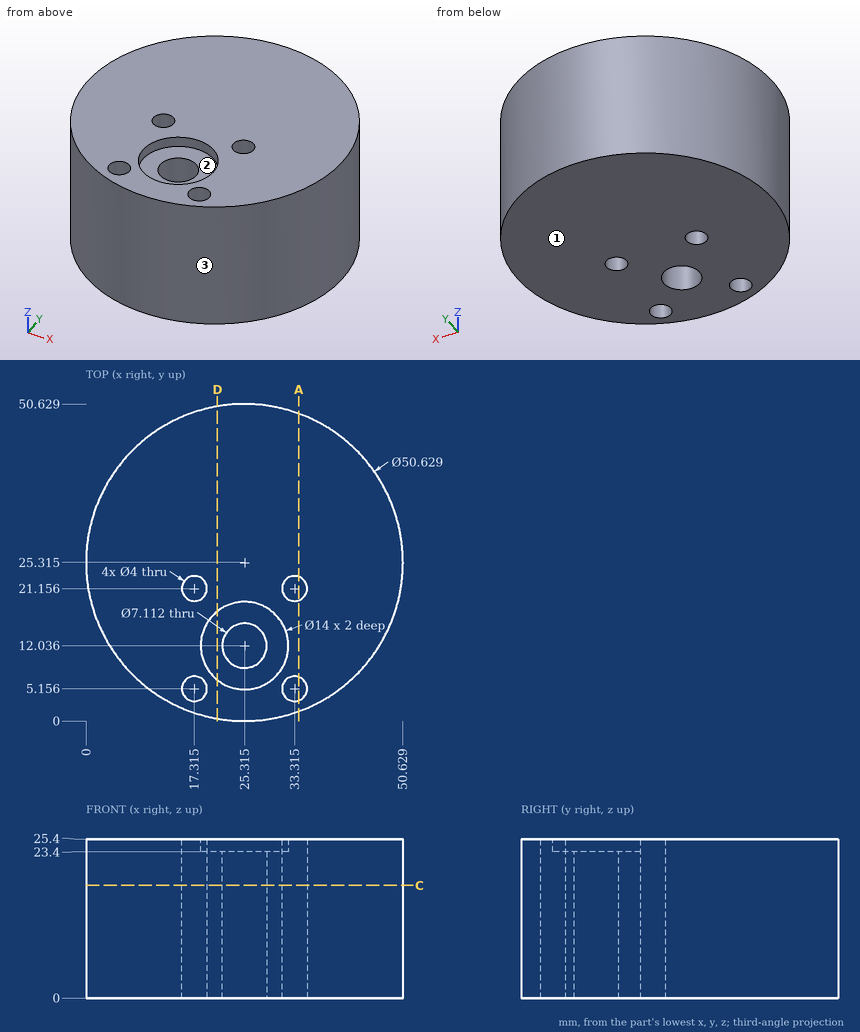
Verification items for this drawing (mm, ordinates from the low corner). Round coordinates to 2 decimals unless told otherwise and drop trailing zeros. Write each loop counter-clockwise with the first axis right and the second up, starting at its lowest first coordinate (ties: lowest second). Pieces come first, ordered by that corner, then holes. Notation, with made-up numbers: (58, -36) - (96, -36) arc R11 cw to (96, -17) - close; hole circle Ø3 at (61, -36.5). An arc over 180 degrees is marked (long way). Answer as a JSON object with one key per item and string values. Group by question number.
Q1. Go/stop test with flat-tipped pins: pin 1 Ø22.5 at (x, y) = (25.31, 12.04) entering from +Z; pin 2 Ø3 at (x, z) = (34.5, 22.5) entering from -Y (1 decimal); pin 3 Ø1.5 at (x, z) = (18.5, 16.5) entering from -Y; pin 4 Ø1 at (y, z) = (33.5, 4.5) entering from -X (1 decimal). Record where each tip stops, or that it passes through.
Q2. Thickness scan on line 1 (X direction, y = 5.5, z = 17.75) (1 decimal); line 2 (X direction, y = 26, z = 10.75); line 3 (Z direction, x = 22, y = 8). Record the ranges inside material, lowest first.
Q3. Mould release check, pull along Y, two halves, no side actions. Record for the marked faces 1, 2 and 3: released by +Y, released by -Y, zero draft, split by the parting line, or undercut.
Q4. Section check A-A, the plane x = 34. Enter the section's corners in (y, z) (1 decimal), plus the area to 3 significant figures.
Q5. Section check C-C, the plane z = 18. Enter the section's corners in (x, y) (1 decimal), plus the area to 3 significant figures.
Q6. Section check D-D, the plane x = 21. Enter the section's corners in (y, z).
Found:
{
 "1": {"pin 1": "stops at z = 25.4", "pin 2": "stops at y = 1.2", "pin 3": "stops at y = 0.74", "pin 4": "stops at x = 1.2"},
 "2": {"line 1": "x = 9.6 to 15.3, 19.3 to 31.3, 35.3 to 41.1", "line 2": "x = 0.01 to 50.62", "line 3": "z = 0 to 23.4"},
 "3": {"face 1": "zero draft", "face 2": "undercut", "face 3": "split by the parting line"},
 "4": {"outline": "(1.5, 0) - (3.3, 0) - (3.3, 25.4) - (1.5, 25.4) - close; (7, 0) - (19.3, 0) - (19.3, 25.4) - (7, 25.4) - close; (23, 0) - (49.1, 0) - (49.1, 25.4) - (23, 25.4) - close", "area": "1,020 mm^2"},
 "5": {"outline": "circle Ø50.6 at (25.3, 25.3); hole circle Ø4 at (17.3, 5.2); hole circle Ø4 at (17.3, 21.2); hole circle Ø7.1 at (25.3, 12); hole circle Ø4 at (33.3, 5.2); hole circle Ø4 at (33.3, 21.2)", "area": "1,920 mm^2"},
 "6": {"outline": "(0.37, 0) - (50.26, 0) - (50.26, 25.4) - (17.55, 25.4) - (17.55, 23.4) - (6.52, 23.4) - (6.52, 25.4) - (0.37, 25.4) - close"}
}
